Work out the finished part from the listing and answer in its coordinate system (mm). Coordinates: 2 decimals unless noted, no trailing zeros. Order: outer loops, then holes, each group sorted by start corner. A loop starts at its lowest first (then second) coordinate and runs counter-clockwise, first axis right, second up. Notation, with made-up numbers: (35, -39) - (61, -39) arc R24 ccw to (61, -25) - close; hole circle Ø6 at (21, 22.5). An arc over 180 degrees is marked (long way). Answer as a JSON object with one key per item and string values. Group by question number.
1) Each of these flat-tipped pins is pushed along its axis until it touches: P1, Ø2.5, axis at x = -4.88, z = 43.99, coming from the -Y side; P2, Ø1.5, axis at y = -2, z = 18.5, coming from the -X side. Where does it stop, or does it pass through?
2) The mould has two halves that part along X. Classify faces 1 (the face through (-47.794, -1.479, 2.512)), 2 (the face through (-5.141, -1.479, 45.975)), 3 (the face through (-19, -3, 19)), 4 (the face through (-1.256, -1.479, 1.168)): released by +X, released by -X, zero draft, split by the parting line, or undercut.
3) Section B-B (x = -16) is taken. Give the vertices of the cut face in (y, z).
4) Find the intervals of material crossed by line 1 along Z through (x, y) = (-3.5, -0.5); line 2 along Z through (x, y) = (-44, -0.5); line 3 along Z through (x, y) = (-5, -1.1), in increasing order.
5) Section A-A (y = -2.1) is taken. Give the vertices of the cut face in (x, z), plus the area to 3 significant figures.
6) Section C-C (z = 14.5) is taken. Give the vertices of the cut face in (x, y), plus the area to 3 significant figures.
from build123d import *

# Parameters (mm, degrees)
F0_R     = 2
F1_DEPTH = 3


with BuildPart() as f1:
    # F0 (on Front) → F1 (new body)
    with BuildSketch(Plane.XZ):
        with BuildLine():
            ThreePointArc((-4.080816, 0), (-1.224245, 1.2), (-0.081616, 4.08))
            Line((-0.081616, 4.08), (-0.881616, 44.071999))
            ThreePointArc((-0.881616, 44.071999), (-3.405689, 47.710063), (-7.737388, 46.791999))
            Line((-7.737388, 46.791999), (-46.937388, 6.8))
            ThreePointArc((-46.937388, 6.8), (-47.768634, 2.450807), (-44.080816, 0))
            Line((-44.080816, 0), (-4.080816, 0))
        make_face()
        with Locations((-44.080816, 4)):
            Circle(F0_R, mode=Mode.SUBTRACT)
        with Locations((-4.080816, 4)):
            Circle(F0_R, mode=Mode.SUBTRACT)
        with Locations((-4.880816, 43.991999)):
            Circle(F0_R, mode=Mode.SUBTRACT)
    extrude(amount=F1_DEPTH)


solid = f1.part
Report:
{
 "1": {"P1": "passes through", "P2": "stops at x = -36.2"},
 "2": {"face 1": "released by -X", "face 2": "undercut", "face 3": "zero draft", "face 4": "released by +X"},
 "3": {"outline": "(-3, 0) - (0, 0) - (0, 38.36) - (-3, 38.36) - close"},
 "4": {"line 1": "z = 0.04 to 2.09, 5.91 to 42.55, 45.44 to 47.75", "line 2": "z = 0 to 2, 6 to 9.8", "line 3": "z = 0 to 2.22, 5.78 to 42, 45.99 to 47.99"},
 "5": {"outline": "(-46.94, 6.8) arc R4 ccw to (-44.08, 0) - (-4.08, 0) arc R4 ccw to (-0.08, 4.08) - (-0.88, 44.07) arc R4 ccw to (-7.74, 46.79) - close; hole circle Ø4 at (-44.08, 4); hole circle Ø4 at (-4.88, 43.99); hole circle Ø4 at (-4.08, 4)", "area": "1,360 mm²"},
 "6": {"outline": "(-39.39, -3) - (-0.29, -3) - (-0.29, 0) - (-39.39, 0) - close", "area": "117 mm²"}
}
